Autodesk Inventor part; units mm, degrees
ref_plane "YZ Plane" through (0, 0, 0) normal (1, 0, 0) x (0, 1, 0)
ref_plane "XZ Plane" through (0, 0, 0) normal (0, 1, 0) x (-1, 0, 0)
ref_plane "XY Plane" through (0, 0, 0) normal (0, 0, 1) x (1, 0, 0)
sketch "Sketch1" plane through (0, 0, 0) normal (0, 1, 0) x (-1, 0, 0)
  line L0 (-280, 300) -> (280, 300)
  line L1 (300, 280) -> (300, -280)
  line L2 (280, -300) -> (-280, -300)
  line L3 (-300, -280) -> (-300, 280)
  line L4 (-300, 300) -> (300, -300) construction
  line L5 (300, 300) -> (-300, -300) construction
  arc A0 (300, 280) -> (280, 300) centre (280, 280) ccw
  arc A1 (280, -300) -> (300, -280) centre (280, -280) ccw
  arc A2 (-300, -280) -> (-280, -300) centre (-280, -280) ccw
  arc A3 (-280, 300) -> (-300, 280) centre (-280, 280) ccw
  line L6 (280, 294) -> (-280, 294)
  arc A4 (-280, 294) -> (-294, 280) centre (-280, 280) ccw
  line L7 (-294, 280) -> (-294, -280)
  arc A5 (-294, -280) -> (-280, -294) centre (-280, -280) ccw
  line L8 (-280, -294) -> (280, -294)
  arc A6 (280, -294) -> (294, -280) centre (280, -280) ccw
  line L9 (294, -280) -> (294, 280)
  arc A7 (294, 280) -> (280, 294) centre (280, 280) ccw
  point P0 (0, 0)
  dimension "d0" = 600
  dimension "d1" = 600
  dimension "d2" = 20
  dimension "d3" = 6
extrude "Extrusion1" add sketch "Sketch1" along normal blind 300
properties part number "Stackbox-noHoles"
Geometry: final body of the model. Coordinates: model frame, mm. A direction names the side the tool comes from. Round coordinates to 2 decimals unless told otherwise and drop trailing zeros. Write each loop counter-clockwise with the first axis right and the second up, starting at its lowest first coordinate (ties: lowest second). Pieces come first, ordered by that corner, then holes. Notation, with made-up numbers: M 39.25,55.25 L 65.25,55.25 A20 cw 65.25,65.25 Z; hole C 54.25,39.25 d10. An arc over 180 degrees is marked long. Answer in a Markdown table with one row per item. Add a question column.
(1) Ray query, L1, parallel to X at y = 53.5, z = 12. Return the intervals inside material, ascending.
(2) Reachability of faces 5 (the face through (294, 148, 4)), 6 (the face through (-4, 148, -300)) from +Z, -Z, +X, -X, +Y, -Y: full face, straight path, thin tool, end or side. Return the list, or none.
(3) Cut plane A-A, the plane z = -52.5. Return the cut outline in (x, y).
(4) Draft query along Z for faces 1 (the face through (4, 148, 300)), 2 (the face through (300, 148, -4)), 3 (the face through (-294.297, 147.9, -293.986)), 4 (the face through (-289.8, 147.9, 290)). Return one class per face: pulls with the +Z half, pulls with the -Z half, needs draft (parallel to the pull), parting line crosses it, or undercut.
(5) Cut plane B-B, the plane x = 240.5. Return the cut outline in (y, z).
(6) Cut plane C-C, the plane y = 62.5. Return the cut outline in (x, z), then the cut area to 3 significant figures.
Established:
| question | item | result |
|---|---|---|
| 1 | L1 | -300 to -294, 294 to 300 |
| 2 | face 5 | +Y, -Y |
| 2 | face 6 | -Z, +X, -X, +Y, -Y |
| 3 | outline | M -300,0 L -294,0 L -294,300 L -300,300 Z; M 294,0 L 300,0 L 300,300 L 294,300 Z |
| 4 | face 1 | pulls with the +Z half |
| 4 | face 2 | needs draft |
| 4 | face 3 | pulls with the -Z half |
| 4 | face 4 | undercut |
| 5 | outline | M 0,-300 L 300,-300 L 300,-294 L 0,-294 Z; M 0,294 L 300,294 L 300,300 L 0,300 Z |
| 6 | outline | M -300,-280 A20 ccw -280,-300 L 280,-300 A20 ccw 300,-280 L 300,280 A20 ccw 280,300 L -280,300 A20 ccw -300,280 Z; hole M -294,-280 A14 ccw -280,-294 L 280,-294 A14 ccw 294,-280 L 294,280 A14 ccw 280,294 L -280,294 A14 ccw -294,280 Z |
| 6 | area | 14,100 mm² |
